from build123d import *

# Parameters (mm, degrees)
SKETCH1_W           = 28
SKETCH1_H           = 56.5
BOSS_EXTRUDE1_DEPTH = 30
CUT_EXTRUDE2_DEPTH  = 56.5
SHELL1_T            = -1
BOSS_EXTRUDE3_DEPTH = 2.5
SKETCH4_R           = 0.35
CUT_EXTRUDE1_DEPTH  = 5
BOSS_EXTRUDE4_DEPTH = 56.5
BOSS_EXTRUDE5_START = -11.087816
SKETCH7_R           = 8.5
BOSS_EXTRUDE5_DEPTH = 11.087816
SKETCH8_R           = 7
CUT_EXTRUDE3_DEPTH  = 2
LPATTERN1_COUNT     = 2
LPATTERN1_PITCH     = 20


with BuildPart() as part:
    # Sketch1 → Boss-Extrude1 (new body)
    with BuildSketch(Plane(origin=(0, 0, 0), x_dir=(1, 0, 0), z_dir=(0, 1, 0))):
        Rectangle(SKETCH1_W, SKETCH1_H)
    extrude(amount=-BOSS_EXTRUDE1_DEPTH)

    # Sketch5 → Cut-Extrude2 (cut)
    with BuildSketch(Plane(origin=(0, 0, -28.25), x_dir=(-1, 0, 0), z_dir=(0, 0, -1))):
        with BuildLine():
            Line((-1, -30), (-1, -26))
            ThreePointArc((-1, -26), (3.188611699, -13.752551286), (14, -6.635083269))
            Line((14, -6.635083269), (14, -30))
            Line((14, -30), (-1, -30))
        make_face()
    extrude(amount=-CUT_EXTRUDE2_DEPTH, mode=Mode.SUBTRACT)

    # Shell1
    shell1_openings = [part.faces().sort_by_distance(p)[0] for p in [
        (7.5, -30, 0),
        (0.885231383, -15.011682153, 28.25),
        (-14, -3.317541634, 0),
        (-4.84430585, -15.03504646, 0),
        (1, -28, 0),
    ]]
    offset(amount=SHELL1_T, openings=shell1_openings, kind=Kind.INTERSECTION)

    # Sketch3 → Boss-Extrude3 (add, symmetric)
    with BuildSketch(Plane.XY.offset(-20)):
        with BuildLine():
            Line((-14, -1), (-15, -1))
            ThreePointArc((-15, -1), (-15.5, -1.5), (-15, -2))
            Line((-15, -2), (-14, -2))
            Line((-14, -2), (-12.5, -1))
            Line((-12.5, -1), (-14, -1))
        make_face()
    boss_extrude3 = extrude(amount=BOSS_EXTRUDE3_DEPTH, both=True)

    # Sketch4 → Cut-Extrude1 (cut)
    with BuildSketch(Plane(origin=(0, 0, -22.5), x_dir=(-1, 0, 0), z_dir=(0, 0, -1))):
        with Locations((15, -1.5)):
            Circle(SKETCH4_R)
    cut_extrude1 = extrude(amount=-CUT_EXTRUDE1_DEPTH, mode=Mode.SUBTRACT)

    # Mirror1: Boss-Extrude3, Cut-Extrude1 across plane
    add(boss_extrude3.mirror(Plane.XY))
    add(cut_extrude1.mirror(Plane.XY), mode=Mode.SUBTRACT)

    # Sketch6 → Boss-Extrude4 (add)
    with BuildSketch(Plane(origin=(0, 0, -28.25), x_dir=(-1, 0, 0), z_dir=(0, 0, -1))):
        Polygon((-30, -3.677832944), (-21, -25), (-14, -30), (-14, 0), align=None)
        with BuildLine():
            Line((14, 0), (14, 2.5))
            ThreePointArc((14, 2.5), (-0.085690207, 2.209730318), (-14, 0))
            Line((-14, 0), (14, 0))
        make_face()
    extrude(amount=-BOSS_EXTRUDE4_DEPTH)

    # Sketch7 → Boss-Extrude5 (add)
    with BuildSketch(Plane(origin=(33, 0, 0), x_dir=(0, 0, -1), z_dir=(1, 0, 0)).offset(BOSS_EXTRUDE5_START)):
        with Locations((10.25, -14.338916472)):
            Circle(SKETCH7_R)
    boss_extrude5 = extrude(amount=BOSS_EXTRUDE5_DEPTH)

    # Sketch8 → Cut-Extrude3 (cut)
    with BuildSketch(Plane(origin=(33, 0, 0), x_dir=(0, 0, -1), z_dir=(1, 0, 0))):
        with Locations((10.25, -14.338916472)):
            Circle(SKETCH8_R)
    cut_extrude3 = extrude(amount=-CUT_EXTRUDE3_DEPTH, mode=Mode.SUBTRACT)

    # LPattern1: Boss-Extrude5, Cut-Extrude3 ×2
    with Locations(*[(0, 0, i * LPATTERN1_PITCH) for i in range(1, LPATTERN1_COUNT)]):
        add(boss_extrude5)
        add(cut_extrude3, mode=Mode.SUBTRACT)


solid = part.part
The model under review builds one solid part; all positions refer to its coordinate system, in mm. A direction names the side the tool comes from. Round coordinates to 2 decimals unless told otherwise and drop trailing zeros. Loops run counter-clockwise (first coordinate to the right, second up) from the corner with the lowest first, then second, coordinate; pieces in that order, holes last. Notation, with made-up numbers: M 40.5,27.5 L 49.5,27.5 A4 cw 49.5,32.5 Z; hole C -15.75,-33 d9. An arc over 180 degrees is marked long. Answer as CSV lines item,"result". Start each with the question number.
Item 1: Consider section B-B (y = -22). Write out the cut boundary in (x, z), then the cut area to 3 significant figures.
Item 2: Insertion check: P1, Ø0.5, axis at x = -14, y = -1.5, coming from the +Z side; P2, Ø12, axis at x = 28, y = -12.5, coming from the +Z side; P3, Ø1, axis at x = -10.5, z = 10, coming from the +Y side; P4, Ø5, axis at x = -3.5, y = -20, coming from the +Z side. Each pin has a flat end and moves straight along its axis. Give the tip position at first contact, or say it passes through.
Item 3: For faces 1 (the face through (-13.26, -1.507, -19.965)), 2 (the face through (21.888, -1.813, -0.396)), 3 (the face through (31, -14, 10)), list the 3-axis set-ups (+Z, -Z, +X, -X, +Y, -Y) from which the entire face can be reached by the end or side of a thin tool; tool diameter is ignored.
Item 4: Wall thickness on line 1 (Y direction, x = 31.8, z = 9.75); line 2 (Y direction, x = -15, z = -18); line 3 (Z direction, x = 8.5, y = -4): over which ranges is each line inside the solid? List them lowest first. Write a range as [from, to].
Item 5: Consider section C-C (x = -6.5). Write out the cut boundary in (y, z), then the cut area to 3 significant figures.
Item 6: Mouldability with a two-part tool opening along X and no side actions: class faces 4 (the face through (32.014, -8.436, 5.987)), 5 (the face through (-13.26, -1.507, 19.965)), 6 (the face through (17.5, -27.5, -0.4)) as released by +X, released by -X, zero draft, split by the parting line, or undercut.
Item 7: Consider section D-D (z = 9.75). Write out the cut boundary in (x, y), then the cut area to 3 significant figures.
Item 8: Consider section A-A (z = 24.5). Write out the cut boundary in (x, y), then the cut area to 3 significant figures.
Answer:
1,outline,"M 0.6,-28.25 L 22.27,-28.25 L 22.27,-13.93 L 33,-13.93 L 33,-6.57 L 22.27,-6.57 L 22.27,6.07 L 33,6.07 L 33,13.43 L 22.27,13.43 L 22.27,28.25 L 13,28.25 L 13,-27.25 L 0.6,-27.25 Z"
1,area,"694 mm^2"
2,P1,"stops at z = 22.5"
2,P2,"stops at z = 28.25"
2,P3,"stops at y = 2.61"
2,P4,"passes through"
3,face 1,"+Z, -Y"
3,face 2,"+Z, -Z, +X, +Y"
3,face 3,"+X"
4,line 1,"y = [-22.84, -21.34], [-7.34, -5.84]"
4,line 2,"y = [-2, -1.85], [-1.15, -1]"
4,line 3,"z = [-28.25, -27.25]"
5,outline,"M -10.39,-28.25 L 2.59,-28.25 L 2.59,28.25 L -1,28.25 L -1,-27.25 L -10.39,-27.25 Z"
5,area,"212 mm^2"
6,face 4,"zero draft"
6,face 5,"undercut"
6,face 6,"released by +X"
7,outline,"M -14,-1 L 13,-1 L 13,-30 L 14,-30 L 21,-25 L 21.91,-22.84 L 33,-22.84 L 33,-21.34 L 31,-21.34 L 31,-7.34 L 33,-7.34 L 33,-5.84 L 29.09,-5.84 L 30,-3.68 L 14,0 A103 ccw -14,2.5 Z"
7,area,"502 mm^2"
8,outline,"M -14,-1 L 13,-1 L 13,-30 L 14,-30 L 21,-25 L 30,-3.68 L 14,0 A103 ccw -14,2.5 Z"
8,area,"402 mm^2"
